Work out the finished part from the listing and answer in its coordinate system (mm). Face numbers are marked on the shaded views. Round coordinates to 2 decimals unless told otherwise and drop trailing zeros. Order: outer loops, then holes, each group sorted by start corner. A loop starts at its lowest first (then second) coordinate and runs counter-clockwise, first axis right, second up. Notation, with made-up numbers: M 58,-36.5 L 93,-36.5 A27 ccw 93,-7.5 Z; hole C -6.75,2.5 d11. An arc over 180 degrees is marked long. Return JSON: item names as keys, results as strings.
from build123d import *

# Parameters (mm, degrees)
SKETCH1_W                                        = 23
SKETCH1_H                                        = 50
BOSS_EXTRUDE1_DEPTH                              = 4
M4_CLEARANCE_HOLE1_D                             = 4.5
FILLET1_R                                        = 3
SKETCH4_R                                        = 3
CUT_EXTRUDE1_DEPTH                               = 10
CBORE_FOR_M2_PAN_HEAD_MACHINE_SCREW1_D           = 2.4
CBORE_FOR_M2_PAN_HEAD_MACHINE_SCREW1_CBORE_D     = 5
CBORE_FOR_M2_PAN_HEAD_MACHINE_SCREW1_CBORE_DEPTH = 1.6


with BuildPart() as part:
    # Sketch1 → Boss-Extrude1 (new body)
    with BuildSketch(Plane(origin=(0, 0, 0), x_dir=(1, 0, 0), z_dir=(0, 1, 0))):
        Rectangle(SKETCH1_W, SKETCH1_H)
    extrude(amount=BOSS_EXTRUDE1_DEPTH)

    # M4 Clearance Hole1 (through all)
    with Locations(Plane(origin=(0, 4, 0), x_dir=(1, 0, 0), z_dir=(0, 1, 0))):
        with Locations((-7.5, 20), (7.5, 20), (-7.5, -20), (7.5, -20)):
            Hole(M4_CLEARANCE_HOLE1_D / 2)

    # Fillet1
    fillet1_edges = [part.edges().sort_by_distance(p)[0] for p in [
        (11.5, 2, 25),
        (-11.5, 2, 25),
        (-11.5, 2, -25),
        (11.5, 2, -25),
    ]]
    fillet(fillet1_edges, radius=FILLET1_R)

    # Sketch4 → Cut-Extrude1 (cut)
    with BuildSketch(Plane(origin=(0, 0, 0), x_dir=(1, 0, 0), z_dir=(0, 1, 0))):
        with Locations(Location((0, 0, 0), (0, 0, 90))):
            Circle(SKETCH4_R)
    extrude(amount=CUT_EXTRUDE1_DEPTH, mode=Mode.SUBTRACT)

    # CBORE for M2 Pan Head Machine Screw1 (through all)
    with Locations(Plane(origin=(0, 0, 0), x_dir=(-1, 0, 0), z_dir=(0, -1, 0))):
        with Locations((0, -8), (-6, 0), (0, 8), (6, 0)):
            CounterBoreHole(CBORE_FOR_M2_PAN_HEAD_MACHINE_SCREW1_D / 2, CBORE_FOR_M2_PAN_HEAD_MACHINE_SCREW1_CBORE_D / 2, CBORE_FOR_M2_PAN_HEAD_MACHINE_SCREW1_CBORE_DEPTH)


solid = part.part
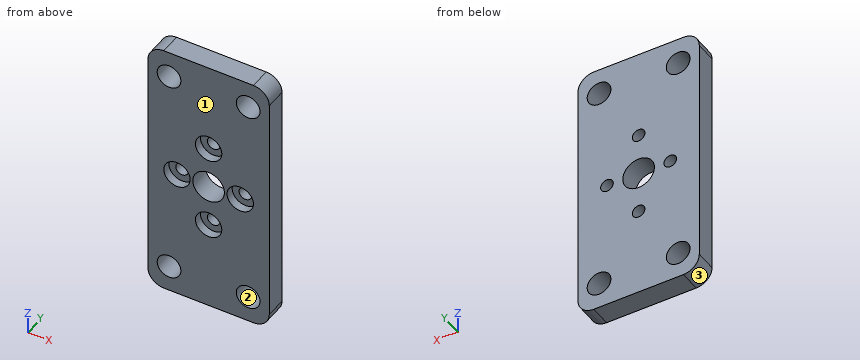
Item 1: The mould has two halves that part along Z. Classify the marked faces 1, 2 and 3: pulls with the +Z half, pulls with the -Z half, needs draft (parallel to the pull), parting line crosses it, or undercut.
Output:
{"face 1": "needs draft", "face 2": "undercut", "face 3": "pulls with the -Z half"}
Item 2: Find section B-B (x = 0). Determine the outline of the cut face in (y, z), plus the area to 3 significant figures.
Output:
{"outline": "M 0,-25 L 4,-25 L 4,-9.2 L 1.6,-9.2 L 1.6,-10.5 L 0,-10.5 Z; M 0,-5.5 L 1.6,-5.5 L 1.6,-6.8 L 4,-6.8 L 4,-3 L 0,-3 Z; M 0,3 L 4,3 L 4,6.8 L 1.6,6.8 L 1.6,5.5 L 0,5.5 Z; M 0,10.5 L 1.6,10.5 L 1.6,9.2 L 4,9.2 L 4,25 L 0,25 Z", "area": "148 mm^2"}
Item 3: Each of these flat-tipped pins is pushed along its axis until it touches: pin 1 (1.5 mm diameter, centred on x = 1, z = 9, fed in from -Y); pin 2 (6.5 mm diameter, centred on x = -6, z = 0, fed in from -Y); pin 3 (2.5 mm diameter, centred on x = 7.5, z = 20, fed in from -Y). Where does it stop, or does it pass through?
Output:
{"pin 1": "stops at y = 1.6", "pin 2": "stops at y = 0", "pin 3": "passes through"}
Item 4: Find section D-D (z = -20). Determine the outline of the cut face in (x, y).
Output:
{"outline": "M -11.5,0 L -9.75,0 L -9.75,4 L -11.5,4 Z; M -5.25,0 L 5.25,0 L 5.25,4 L -5.25,4 Z; M 9.75,0 L 11.5,0 L 11.5,4 L 9.75,4 Z"}
Item 5: Find section C-C (y = 2.1). State how many separate pieces and enclosed holes the cut face has, plus the area to 3 significant figures.
Output:
{"separate pieces": "1", "enclosed holes": "9", "area": "1,030 mm^2"}
Item 6: Consider line 1 along Z through (x, y) = (7.5, 2.95); line 2 along X through (y, z) = (1.2, 20); line 3 along X through (y, z) = (0.45, 8). Determine where each line is inside the solid, lowest interval first. Write a range as [from, to].
Output:
{"line 1": "z = [-25, -22.25], [-17.75, 17.75], [22.25, 25]", "line 2": "x = [-11.5, -9.75], [-5.25, 5.25], [9.75, 11.5]", "line 3": "x = [-11.5, -2.5], [2.5, 11.5]"}
Item 7: Find section A-A (z = 0). Determine the outline of the cut face in (x, y).
Output:
{"outline": "M -11.5,0 L -8.5,0 L -8.5,1.6 L -7.2,1.6 L -7.2,4 L -11.5,4 Z; M -4.8,1.6 L -3.5,1.6 L -3.5,0 L -3,0 L -3,4 L -4.8,4 Z; M 3,0 L 3.5,0 L 3.5,1.6 L 4.8,1.6 L 4.8,4 L 3,4 Z; M 7.2,1.6 L 8.5,1.6 L 8.5,0 L 11.5,0 L 11.5,4 L 7.2,4 Z"}
